Design review of the part shown in the three views and the two pictorial views. Dimensions are in mm from the part's minimum x, y and z. Round coordinates to 2 decimals unless told otherwise and drop trailing zeros. Order: outer loops, then holes, each group sorted by start corner. A loop starts at its lowest first (then second) coordinate and runs counter-clockwise, first axis right, second up. Notation, with made-up numbers: M 7.5,48.5 L 30.5,48.5 A29 cw 30.5,83.5 Z; hole C -20,-25 d10. An arc over 180 degrees is marked long. Use a Markdown table: item, result. Add a question column.
(1) For pin 1 (0.5 mm diameter, centred on x = 112.5, z = 22.5, fed in from -Y); pin 2 (8 mm diameter, centred on y = 17.5, z = 32.5, fed in from -X) (1 decimal); pin 3 (10 mm diameter, centred on y = 7, z = 19, fed in from -X); pin 4 (5 mm diameter, centred on x = 56.5, z = 25, fed in from -Y), all flat-tipped, find the tip position at first contact; note any pin that passes through.
(2) Take a section at D-D (z = 35.5). Write out the cut boundary in (x, y) (1 decimal).
(3) Take a section at B-B (y = 21.75). Write out the cut boundary in (x, z) (1 decimal).
(4) Take a section at C-C (z = 26.7). Write out the cut boundary in (x, y) (1 decimal).
(5) To check wall thickness, follow probe 1 along Z at (x, y) = (95.5, 23.5); probe 2 along Z at (x, y) = (58.5, 15.5); probe 3 along X at (y, z) = (21.75, 26.7) (1 decimal). State the ranges of each line that lie inside material, in increasing order. Write a range as from..to.
(6) The part is to be moulded in two halves that separate along Z. For the marked faces 1, 2, 3 and 4, say which applies: released by +Z, released by -Z, zero draft, split by the parting line, or undercut.
(7) Take a section at A-A (x = 49). Write out the cut boundary in (y, z).
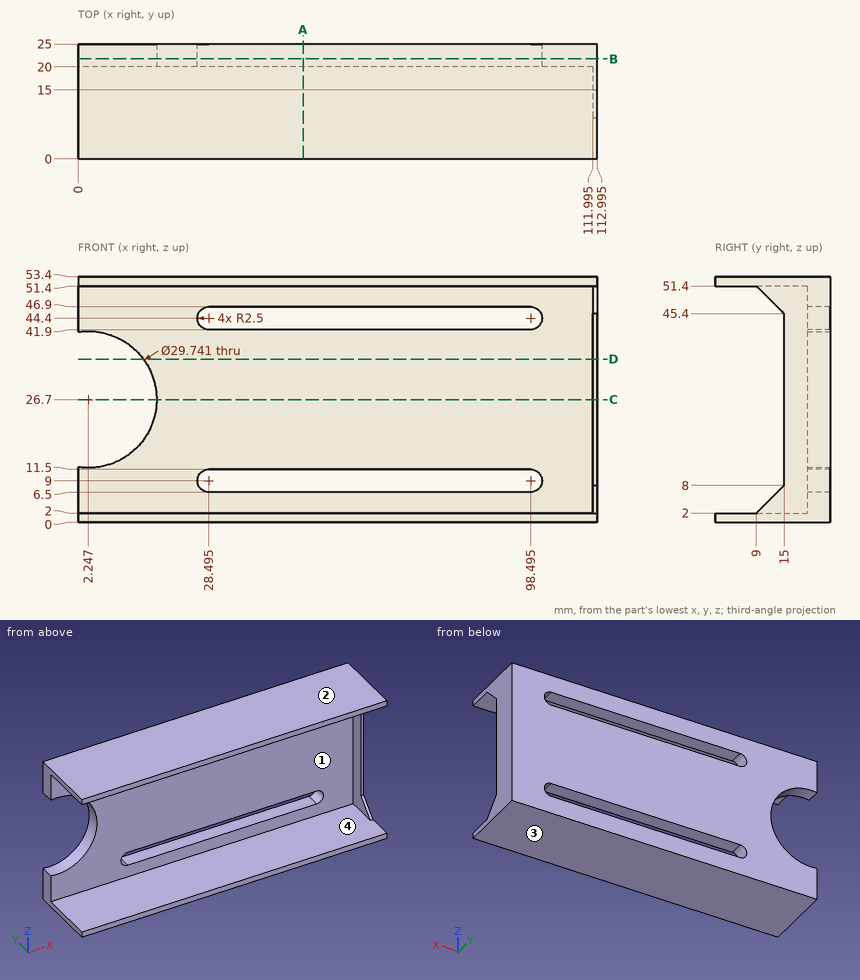
Verdict:
| question | item | result |
|---|---|---|
| 1 | pin 1 | stops at y = 15 |
| 1 | pin 2 | stops at x = 14.1 |
| 1 | pin 3 | passes through |
| 1 | pin 4 | stops at y = 20 |
| 2 | outline | M 14.2,20 L 112,20 L 112,15 L 113,15 L 113,25 L 14.2,25 Z |
| 3 | outline | M 0,0 L 113,0 L 113,53.4 L 0,53.4 L 0,41.4 A14.9 cw long 0,12 Z; hole M 28.5,6.5 L 98.5,6.5 A2.5 ccw 98.5,11.5 L 28.5,11.5 A2.5 ccw Z; hole M 28.5,41.9 L 98.5,41.9 A2.5 ccw 98.5,46.9 L 28.5,46.9 A2.5 ccw Z |
| 4 | outline | M 17.1,20 L 112,20 L 112,15 L 113,15 L 113,25 L 17.1,25 Z |
| 5 | probe 1 | z = 0..6.5, 11.5..41.9, 46.9..53.4 |
| 5 | probe 2 | z = 0..2, 51.4..53.4 |
| 5 | probe 3 | x = 17.1..113 |
| 6 | face 1 | undercut |
| 6 | face 2 | released by +Z |
| 6 | face 3 | released by -Z |
| 6 | face 4 | undercut |
| 7 | outline | M 0,0 L 25,0 L 25,6.5 L 20,6.5 L 20,2 L 0,2 Z; M 0,51.4 L 20,51.4 L 20,46.9 L 25,46.9 L 25,53.4 L 0,53.4 Z; M 20,11.5 L 25,11.5 L 25,41.9 L 20,41.9 Z |
